Could you check a few things on this model? Use its own coordinates, in mm. A direction names the side the tool comes from. Give positions to 0.01 mm unless a question says otherwise; leave off trailing zeros. Loops run counter-clockwise (first coordinate to the right, second up) from the corner with the lowest first, then second, coordinate; pieces in that order, holes last. Notation, with made-up numbers: M -22,68.25 L 18,68.25 A32 cw 18,94.25 Z; hole C -20.5,-25 d3. An arc over 180 degrees is marked long. Return JSON: item names as keys, results as strings. Group by question number.
1. If we mould it in two halves opening along X, with no side actions, what happens to faces 5 (the flat face through (240, 169, 2)), 6 (the flat face through (180, 107, 2)), 7 (the flat face through (121, -5, 2)), 8 (the flat face through (-5, 105, 2))? For each: +X half, -X half, draft (parallel to the pull), parting line (faces both ways), or undercut.
2. Please list where these lines run through material, in increasing order: line 1 (Y direction, x = 114, z = 1.3); line 2 (X direction, y = 142, z = 4.5); line 3 (Y direction, x = 59, z = 1.9).
3. For pin 1 (3 mm diameter, centred on y = 155.5, z = 4.5, fed in from -X); pin 2 (2.5 mm diameter, centred on x = 222.5, z = 3.5, fed in from -Y); pin 3 (2.5 mm diameter, centred on y = -2, z = 2, fed in from +X), each with a flat end and sliding along its axis, tell me the tip position at first contact or that it passes through.
4. If we section it at D-D (x = 230.5): Write out the boundary of the cut face in (y, z), plus the area to 3 significant figures.
5. If we section it at C-C (y = 20): Write out the boundary of the cut face in (x, z), plus the area to 3 significant figures.
6. If we section it at B-B (x = 127.5): Write out the boundary of the cut face in (y, z), plus the area to 3 significant figures.
7. For faces 1 (the flat face through (0, 171, 2)), 2 (the flat face through (35, 0, 2)), 3 (the flat face through (205, 0, 2)), 4 (the flat face through (60, 107, 2)), which set-ups out of +Z, -Z, +X, -X, +Y, -Y let a thin tool reach every point of the face, with its end or its side?
8. If we section it at A-A (z = 0.8): Write out the boundary of the cut face in (x, y).
Autodesk Inventor part; units mm, degrees
ref_plane "YZ Plane" through (0, 0, 0) normal (1, 0, 0) x (0, 1, 0)
ref_plane "XZ Plane" through (0, 0, 0) normal (0, 1, 0) x (-1, 0, 0)
ref_plane "XY Plane" through (0, 0, 0) normal (0, 0, 1) x (1, 0, 0)
sketch "Sketch1" plane through (0, 0, 0) normal (0, 0, 1) x (1, 0, 0)
  line L0 (0, 0) -> (240, 0)
  line L1 (240, 0) -> (240, 210)
  line L2 (240, 210) -> (0, 210)
  line L3 (0, 210) -> (0, 0)
  line L4 (0, 80) -> (-5, 80)
  line L5 (-5, 80) -> (-5, 130)
  line L6 (-5, 130) -> (0, 130)
  line L7 (0, 130) -> (0, 80)
  line L8 (120, 0) -> (120, 210) construction
  line L9 (240, 80) -> (245, 80)
  line L10 (245, 80) -> (245, 130)
  line L11 (245, 130) -> (240, 130)
  line L12 (240, 130) -> (240, 80)
  line L13 (60, 104.7) -> (180, 104.7)
  line L14 (180, 104.7) -> (180, 110)
  line L15 (180, 110) -> (60, 110)
  line L16 (60, 110) -> (60, 104.7)
  line L17 (70, 0) -> (170, 0)
  line L18 (170, 0) -> (170, -5)
  line L19 (170, -5) -> (70, -5)
  line L20 (70, -5) -> (70, 0)
  point P0 (240, 80)
  point P1 (170, 0)
  dimension "d0" = 240
  dimension "d1" = 210
  dimension "d2" = 5
  dimension "d3" = 50
  dimension "d6" = 120
  dimension "d7" = 5.3
  dimension "d10" = 100
  dimension "d11" = 5
  dimension "d12" = 50
extrude "Extrusion1" add sketch "Sketch1" along normal blind 5
properties part number "back"
Answer:
{
 "1": {"face 5": "+X half", "face 6": "undercut", "face 7": "draft", "face 8": "-X half"},
 "2": {"line 1": "y = -5 to 104.7, 110 to 210", "line 2": "x = 0 to 240", "line 3": "y = 0 to 210"},
 "3": {"pin 1": "stops at x = 0", "pin 2": "stops at y = 0", "pin 3": "stops at x = 170"},
 "4": {"outline": "M 0,0 L 210,0 L 210,5 L 0,5 Z", "area": "1,050 mm²"},
 "5": {"outline": "M 0,0 L 240,0 L 240,5 L 0,5 Z", "area": "1,200 mm²"},
 "6": {"outline": "M -5,0 L 104.7,0 L 104.7,5 L -5,5 Z; M 110,0 L 210,0 L 210,5 L 110,5 Z", "area": "1,050 mm²"},
 "7": {"face 1": "+Z, -Z, -X, +Y", "face 2": "+Z, -Z, -X, -Y", "face 3": "+Z, -Z, +X, -Y", "face 4": "+Z, -Z"},
 "8": {"outline": "M -5,80 L 0,80 L 0,0 L 70,0 L 70,-5 L 170,-5 L 170,0 L 240,0 L 240,80 L 245,80 L 245,130 L 240,130 L 240,210 L 0,210 L 0,130 L -5,130 Z; hole M 60,104.7 L 180,104.7 L 180,110 L 60,110 Z"}
}
